```python
from build123d import *

# Parameters (mm, degrees)
F1_DEPTH  = 2
F3_DEPTH  = 8
F5_DEPTH  = 2
F7_DEPTH  = 6
F8_R      = 5
F8_R_2    = 6
F9_DEPTH  = 1
F10_R     = 2.5
F11_R     = 2.5
F12_DEPTH = 3.001


# Not quite as in the source:
# - a feature names something its author has since deleted; it is built from what else it names


with BuildPart() as f1:
    # F0 (on Front) → F1 (new body)
    with BuildSketch(Plane.XZ):
        with BuildLine():
            Line((-36.0815, -20), (36.0815, -20))
            ThreePointArc((36.0815, -20), (56.0815, 0), (36.0815, 20))
            Line((36.0815, 20), (-36.0815, 20))
            ThreePointArc((-36.0815, 20), (-56.0815, 0), (-36.0815, -20))
        make_face()
    extrude(amount=F1_DEPTH)

    # F2 (on face) → F3 (join)
    with BuildSketch(Plane.XZ.offset(2)):
        with BuildLine():
            Line((23.3145, -2.5), (0, -2.5))
            Line((0, -2.5), (-23.3145, -2.5))
            ThreePointArc((-23.3145, -2.5), (-25.2279171618, -2.8806023374), (-26.8500339059, -3.9644660941))
            Line((-26.8500339059, -3.9644660941), (-34.3500339059, -11.4644660941))
            ThreePointArc((-34.3500339059, -11.4644660941), (-35.4338976626, -16.9134171618), (-30.8145, -20))
            Line((-30.8145, -20), (0, -20))
            Line((0, -20), (30.8145, -20))
            ThreePointArc((30.8145, -20), (35.4338976626, -16.9134171618), (34.3500339059, -11.4644660941))
            Line((34.3500339059, -11.4644660941), (26.8500339059, -3.9644660941))
            ThreePointArc((26.8500339059, -3.9644660941), (25.2279171618, -2.8806023374), (23.3145, -2.5))
        make_face()
    extrude(amount=F3_DEPTH)

    # F4 (on face) → F5 (cut)
    with BuildSketch(Plane.XZ.offset(10)):
        with BuildLine():
            Line((-26.1429271247, -4.6715728753), (-33.6429271247, -12.1715728753))
            ThreePointArc((-33.6429271247, -12.1715728753), (-34.51001813, -16.5307337295), (-30.8145, -19))
            Line((-30.8145, -19), (30.8145, -19))
            ThreePointArc((30.8145, -19), (34.51001813, -16.5307337295), (33.6429271247, -12.1715728753))
            Line((33.6429271247, -12.1715728753), (26.1429271247, -4.6715728753))
            ThreePointArc((26.1429271247, -4.6715728753), (24.8452337295, -3.80448187), (23.3145, -3.5))
            Line((23.3145, -3.5), (-23.3145, -3.5))
            ThreePointArc((-23.3145, -3.5), (-24.8452337295, -3.80448187), (-26.1429271247, -4.6715728753))
        make_face()
    extrude(amount=-F5_DEPTH, mode=Mode.SUBTRACT)

    # F6 (on face) → F7 (cut)
    with BuildSketch(Plane.XZ.offset(8)):
        with BuildLine():
            ThreePointArc((30.8145, -18), (33.5861385975, -16.1480502971), (32.9358203436, -12.8786796564))
            Line((32.9358203436, -12.8786796564), (25.4358203436, -5.3786796564))
            ThreePointArc((25.4358203436, -5.3786796564), (24.4625502971, -4.7283614025), (23.3145, -4.5))
            Line((23.3145, -4.5), (-23.3145, -4.5))
            ThreePointArc((-23.3145, -4.5), (-24.4625502971, -4.7283614025), (-25.4358203436, -5.3786796564))
            Line((-25.4358203436, -5.3786796564), (-32.9358203436, -12.8786796564))
            ThreePointArc((-32.9358203436, -12.8786796564), (-33.5861385975, -16.1480502971), (-30.8145, -18))
            Line((-30.8145, -18), (30.8145, -18))
        make_face()
    extrude(amount=-F7_DEPTH, mode=Mode.SUBTRACT)

    # F8 (on face) → F9 (join)
    with BuildSketch(Plane.XZ.offset(2)):
        with Locations((-14.952, 12)):
            Circle(F8_R)
        with Locations((-42.0815, 7.5)):
            Circle(F8_R_2)
        with Locations((14.952, 12)):
            Circle(F8_R)
        with Locations((42.0815, 7.5)):
            Circle(F8_R_2)
    extrude(amount=F9_DEPTH)

    # F10 (on face) + F11 (on face) → F12 (cut, through all)
    with BuildSketch(Plane.XZ.offset(3)):
        with Locations((-14.952, 12)):
            Circle(F10_R)
        with Locations((14.952, 12)):
            Circle(F10_R)
    with BuildSketch(Plane.XZ.offset(3)):
        with Locations((-42.0815, 7.5)):
            Circle(F11_R)
        with Locations((42.0815, 7.5)):
            Circle(F11_R)
    extrude(amount=-F12_DEPTH, mode=Mode.SUBTRACT)


solid = f1.part
```
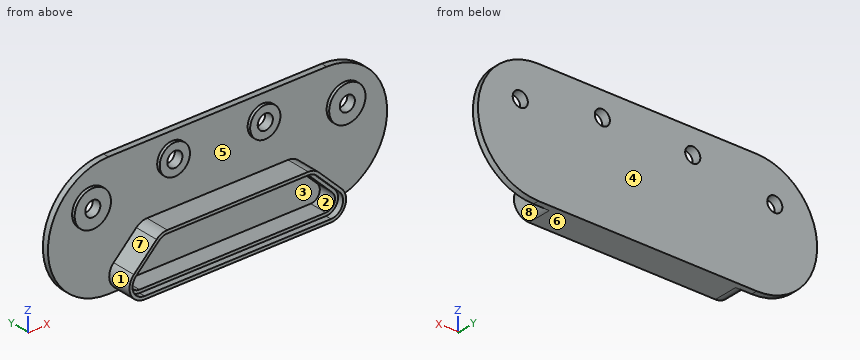
Input: part model. Units: mm. Frame: model coordinates. Face numbers are marked on the shaded views. A direction names the side the tool comes from. Give positions to 0.01 mm unless a question says otherwise; leave off trailing zeros. Order: outer loops, then holes, each group sorted by start corner. A loop starts at its lowest first (then second) coordinate and runs counter-clockwise, first axis right, second up.
1. Reachability of the marked faces 5, 6, 7 and 8 from +Z, -Z, +X, -X, +Y, -Y: full face, straight path, thin tool, end or side. Return the list, or none.
Derived:
face 5: -Y
face 6: -Z, +X, -X, +Y, -Y
face 7: +Z, -X, -Y
face 8: +X, -Y
2. Pin query (flat end, axial travel): pin 1 (10 mm diameter, centred on x = -18.5, z = -13.5, fed in from -Y); pin 2 (7 mm diameter, centred on x = 12, z = -10, fed in from -Y); pin 3 (8 mm diameter, centred on x = 17, z = 10.5, fed in from -Y); pin 4 (4 mm diameter, centred on x = -14.952, z = 12, fed in from -Y). Return the tip coordinate at first contact, or that it passes through.
Derived:
pin 1: stops at y = -8
pin 2: stops at y = -2
pin 3: stops at y = -3
pin 4: passes through
3. Mould query, pull axis Z, two halves, no side actions, for the marked faces 1, 2, 3 and 4. Classes: released by +Z, released by -Z, zero draft, split by the parting line, or undercut.
Derived:
face 1: split by the parting line
face 2: undercut
face 3: undercut
face 4: zero draft
4. Material intervals for L1, parallel to Z at x = -16, y = -9.5; L2, parallel to Z at x = -23, y = -4.75; L3, parallel to Y at x = -27, z = 4.5, sorted ascending.
Derived:
L1: z = -20 to -19, -3.5 to -2.5
L2: z = -20 to -18, -4.5 to -2.5
L3: y = -2 to 0
5. Section A-A on y = -5.5. Return the cut outline in (x, z), and give its area (3 significant figures).
Derived:
outline: (-34.35, -11.46) arc R5 ccw to (-30.81, -20) - (30.81, -20) arc R5 ccw to (34.35, -11.46) - (26.85, -3.96) arc R5 ccw to (23.31, -2.5) - (-23.31, -2.5) arc R5 ccw to (-26.85, -3.96) - close; hole (-32.94, -12.88) arc R3 ccw to (-30.81, -18) - (30.81, -18) arc R3 ccw to (32.94, -12.88) - (25.44, -5.38) arc R3 ccw to (23.31, -4.5) - (-23.31, -4.5) arc R3 ccw to (-25.44, -5.38) - close
area: 309 mm2
6. Section C-C on x = -15.5. Return the cut outline in (y, z), and give its area (3 significant figures).
Derived:
outline: (-10, -20) - (0, -20) - (0, 9.56) - (-3, 9.56) - (-3, 7.03) - (-2, 7.03) - (-2, -2.5) - (-10, -2.5) - (-10, -3.5) - (-8, -3.5) - (-8, -4.5) - (-2, -4.5) - (-2, -18) - (-8, -18) - (-8, -19) - (-10, -19) - close; (-3, 14.44) - (0, 14.44) - (0, 20) - (-2, 20) - (-2, 16.97) - (-3, 16.97) - close
area: 103 mm2
7. Section B-B on z = 12. Return the cut outline in (x, y), and give its area (3 significant figures).
Derived:
outline: (-52.08, -2) - (-46.05, -2) - (-46.05, -3) - (-38.11, -3) - (-38.11, -2) - (-19.95, -2) - (-19.95, -3) - (-17.45, -3) - (-17.45, 0) - (-52.08, 0) - close; (-12.45, -3) - (-9.95, -3) - (-9.95, -2) - (9.95, -2) - (9.95, -3) - (12.45, -3) - (12.45, 0) - (-12.45, 0) - close; (17.45, -3) - (19.95, -3) - (19.95, -2) - (38.11, -2) - (38.11, -3) - (46.05, -3) - (46.05, -2) - (52.08, -2) - (52.08, 0) - (17.45, 0) - close
area: 214 mm2
8. Section D-D on z = 0. Return the cut outline in (x, y).
Derived:
outline: (-56.08, -2) - (56.08, -2) - (56.08, 0) - (-56.08, 0) - close
